Geometry check sheet. Reference: drawing and pictorial views, mm from the part's lowest x, y, z. A direction names the side the tool comes from. Coordinates: 2 decimals unless noted, no trailing zeros. Loops run counter-clockwise (first coordinate to the right, second up) from the corner with the lowest first, then second, coordinate; pieces in that order, holes last. Notation, with made-up numbers: (-1, 14) -> (26, 14) arc R16 cw to (26, 19) -> close; hole circle Ø3 at (-1.75, 41.5). An arc over 180 degrees is marked (long way). Answer as a JSON object with one key per item and string values.
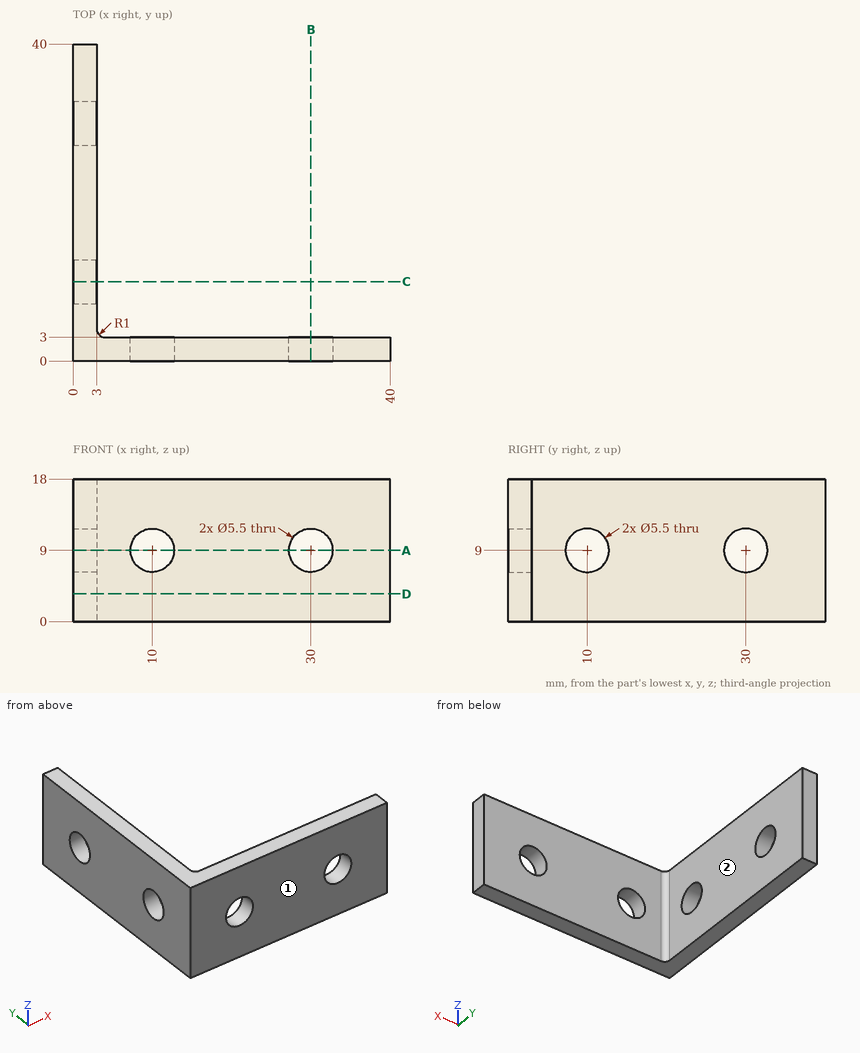
1. Tool access check on the marked faces 1 and 2. Record the directions out of +Z, -Z, +X, -X, +Y, -Y that give a thin tool (end or side, any length) a straight path to the whole face; none if there is none.
Evaluation:
{"face 1": "+Z, -Z, +X, -X, -Y", "face 2": "+Z, -Z, +X, +Y"}
2. Section check B-B, the plane x = 30. Record the boundary of the cut face in (y, z).
Evaluation:
{"outline": "(0, 0) -> (3, 0) -> (3, 6.25) -> (0, 6.25) -> close; (0, 11.75) -> (3, 11.75) -> (3, 18) -> (0, 18) -> close"}
3. Thickness scan on probe 1 along X at (y, z) = (1.85, 9); probe 2 along Z at (x, y) = (30, 1). Record the ranges inside material, lowest first. Write a range as from..to.
Evaluation:
{"probe 1": "x = 0..7.25, 12.75..27.25, 32.75..40", "probe 2": "z = 0..6.25, 11.75..18"}
4. Section check A-A, the plane z = 9. Record the boundary of the cut face in (x, y).
Evaluation:
{"outline": "(0, 0) -> (7.25, 0) -> (7.25, 3) -> (4, 3) arc R1 cw to (3, 4) -> (3, 7.25) -> (0, 7.25) -> close; (0, 12.75) -> (3, 12.75) -> (3, 27.25) -> (0, 27.25) -> close; (0, 32.75) -> (3, 32.75) -> (3, 40) -> (0, 40) -> close; (12.75, 0) -> (27.25, 0) -> (27.25, 3) -> (12.75, 3) -> close; (32.75, 0) -> (40, 0) -> (40, 3) -> (32.75, 3) -> close"}
5. Depth check by flat-ended pin: P1, Ø8, axis at y = 12.5, z = 2.5, coming from the +X side; P2, Ø3, axis at x = 32, z = 6.5, coming from the +Y side. Enter the tip coordinate at first touch or a pass-through.
Evaluation:
{"P1": "stops at x = 3", "P2": "stops at y = 3"}
6. Section check D-D, the plane z = 3.5. Record the boundary of the cut face in (x, y).
Evaluation:
{"outline": "(0, 0) -> (40, 0) -> (40, 3) -> (4, 3) arc R1 cw to (3, 4) -> (3, 40) -> (0, 40) -> close"}
